Autodesk Inventor part; units mm, degrees
ref_plane "YZ Plane" through (0, 0, 0) normal (1, 0, 0) x (0, 1, 0)
ref_plane "XZ Plane" through (0, 0, 0) normal (0, 1, 0) x (-1, 0, 0)
ref_plane "XY Plane" through (0, 0, 0) normal (0, 0, 1) x (1, 0, 0)
sketch "Sketch2" plane through (0, 0, 0) normal (0, 1, 0) x (-1, 0, 0)
  line L0 (0, 0) -> (5, 0)
  line L1 (5, 0) -> (5, -54.829)
  line L2 (5, -54.829) -> (0, -54.829)
  line L3 (0, -54.829) -> (0, 0)
  dimension "d0" = 5
  dimension "d1" = 54.829
extrude "Extrusion1" add sketch "Sketch2" along normal blind 70
sketch "Sketch4" plane through (0, 70, 0) normal (0, 1, 0) x (1, 0, 0)
  line L0 (0, 0) -> (0, 54.829)
  line L1 (0, 54.829) -> (-5, 54.829)
  line L2 (-5, 54.829) -> (-5, 0)
  line L3 (-5, 0) -> (0, 0)
  line L4 (-5, 0) -> (-5, 12.5)
  line L5 (-5, 12.5) -> (0, 12.5)
  line L6 (-5, 12.5) -> (-5, 22.5)
  line L7 (-5, 22.5) -> (0, 22.5)
  line L8 (0, 22.5) -> (0, 32.5)
  line L9 (0, 32.5) -> (-5, 32.5)
  line L10 (-5, 32.5) -> (-5, 42.5)
  line L11 (-5, 42.5) -> (0, 42.5)
  dimension "d8" = 12.5
  dimension "d9" = 10
  dimension "d10" = 10
  dimension "d11" = 10
extrude "Extrusion2" add sketch "Sketch4" along normal blind 5 contours L5 L2 L7 L0 | L9 L2 L11 L0
sketch "Sketch5" plane through (0, 0, 0) normal (0, -1, 0) x (1, 0, 0)
  line L0 (-5, 0) -> (0, 0)
  line L1 (0, 0) -> (0, -54.829)
  line L2 (-5, 0) -> (-5, -12.5)
  line L3 (-5, -12.5) -> (0, -12.5)
  line L4 (-5, -12.5) -> (-5, -22.5)
  line L5 (-5, -22.5) -> (0, -22.5)
  line L6 (-5, -22.5) -> (-5, -32.5)
  line L7 (-5, -32.5) -> (0, -32.5)
  line L8 (-5, -32.5) -> (-5, -42.5)
  line L9 (-5, -42.5) -> (0, -42.5)
  line L10 (-5, -42.5) -> (-5, -54.829)
  line L11 (0, -54.829) -> (-5, -54.829)
  line L12 (0, 0) -> (0, -5.504)
  line L13 (0, -5.504) -> (-5, 0)
  line L14 (0, -54.829) -> (0, -50.141)
  line L15 (0, -50.141) -> (-5, -54.829)
  dimension "d20" = 10
  dimension "d21" = 10
  dimension "d22" = 10
  dimension "d23" = 12.5
  dimension "d24" = 54.829
  dimension "d25" = 12.329
  dimension "d28" = 5.504
  dimension "d29" = 4.688
extrude "Extrusion3" add sketch "Sketch5" along normal blind 5 contours L3 L1 L5 L4 | L7 L1 L9 L8
extrude "Extrusion4" cut sketch "Sketch5" against normal blind 70 contours L0 L1 L13 | L15 L1 L11
sketch "Sketch6" plane through (-5, 70, -12.5) normal (-1, 0, 0) x (0, 0, 1)
  line L0 (-13.5, -70) -> (-15, -70)
  line L1 (-15, -70) -> (-13.5, -70)
  line L2 (-13.5, -70) -> (-15, -70)
  line L3 (-15, -70) -> (-16.5, -70)
  line L4 (-16.5, -70) -> (-15, -70)
  line L5 (-13.5, -70) -> (-13.5, -62)
  line L6 (-13.5, -62) -> (-11.5, -62)
  line L7 (-11.5, -62) -> (-11.5, -57)
  line L8 (-13.5, -70) -> (-16.5, -70)
  line L9 (-16.5, -70) -> (-16.5, -62)
  line L10 (-16.5, -62) -> (-18.5, -62)
  line L11 (-18.5, -62) -> (-18.5, -57)
  line L12 (-18.5, -57) -> (-11.5, -57)
  line L13 (-13.5, 0) -> (-15, 0)
  line L14 (-15, 0) -> (-13.5, 0)
  line L15 (-13.5, 0) -> (-15, 0)
  line L16 (-15, 0) -> (-16.5, 0)
  line L17 (-16.5, 0) -> (-15, 0)
  line L18 (-13.5, 0) -> (-13.5, -8)
  line L19 (-13.5, -8) -> (-11.5, -8)
  line L20 (-11.5, -8) -> (-11.5, -13)
  line L21 (-13.5, 0) -> (-16.5, 0)
  line L22 (-16.5, 0) -> (-16.5, -8)
  line L23 (-16.5, -8) -> (-18.5, -8)
  line L24 (-18.5, -8) -> (-18.5, -13)
  line L25 (-18.5, -13) -> (-11.5, -13)
  point P0 (12.5, -70)
  dimension "d35" = 1.5
  dimension "d36" = 8
  dimension "d37" = 2
  dimension "d38" = 5
  dimension "d39" = 2
extrude "Extrusion5" cut sketch "Sketch6" against normal blind 5
properties part number "lateralnova"
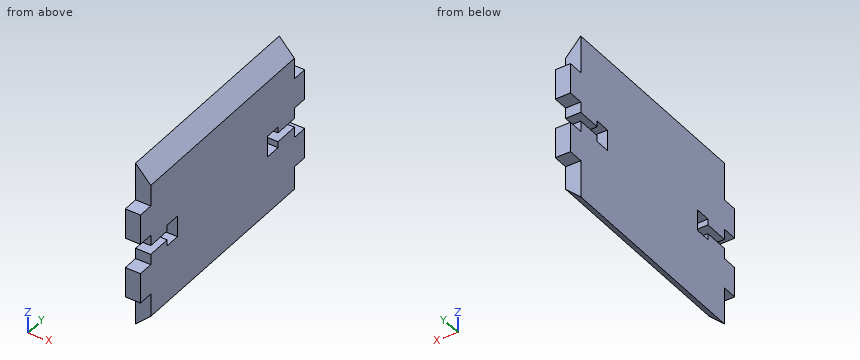
Can you work these out from the model? Positions are in its coordinate system, mm. Coordinates: 2 decimals unless noted, no trailing zeros. Write each loop counter-clockwise with the first axis right and the second up, starting at its lowest first coordinate (ties: lowest second). Pieces come first, ordered by that corner, then holes. Notation, with made-up numbers: (33, -31) -> (60, -31) arc R16 cw to (60, -12) -> close; hole circle Ø11 at (69, -5). An arc over 180 degrees is marked (long way). Write each question's results on one line, items separated by ' | '. Start each with the question number.
Q1. Imagine slicing it at A-A (y = 2). Write out the boundary of the cut face in (x, z), then the cut area to 3 significant figures.
Q2. I'm going to push flat-ended pins straight in: pin 1 (1.5 mm diameter, centred on x = -3.5, y = 72.5, fed in from -Z); pin 2 (2 mm diameter, centred on x = -2, z = -29.5, fed in from +Y); pin 3 (1.5 mm diameter, centred on x = -3.5, z = -4.5, fed in from -Y); pin 4 (5 mm diameter, centred on y = 40, z = -46, fed in from +X). Where does each tip first touch, or does it pass through?
Q3. Imagine slicing it at C-C (y = 50). Write out the boundary of the cut face in (x, z).
Q4. Imagine slicing it at B-B (z = -49). Write out the boundary of the cut face in (x, y).
Q5. If I drill on probe 1 along Y at (x, z) = (-2.8, -30.5); probe 2 along Y at (x, z) = (-3.75, -12); probe 3 along Y at (x, z) = (-3.7, -28), over which ranges is the centre line in solid material (lowest first)?
Taken from the geometry:
1) outline: (-5, -54.83) -> (0, -50.14) -> (0, -29) -> (-5, -29) -> close; (-5, -26) -> (0, -26) -> (0, -5.5) -> (-5, 0) -> close | area: 234 mm^2
2) pin 1: stops at z = -42.5 | pin 2: stops at y = 70 | pin 3: stops at y = 0 | pin 4: stops at x = 0
3) outline: (-5, -54.83) -> (0, -50.14) -> (0, -5.5) -> (-5, 0) -> close
4) outline: (-5, 0) -> (0, 0) -> (0, 70) -> (-5, 70) -> close
5) probe 1: y = 0 to 8, 13 to 57, 62 to 70 | probe 2: y = 0 to 70 | probe 3: y = 13 to 57
